The listing builds one solid part. Answer for the finished solid, in the listing's coordinates (mm). Face numbers are marked on the shaded views. A direction names the side the tool comes from. Round coordinates to 2 decimals unless told otherwise and drop trailing zeros. Write each loop counter-clockwise with the first axis right and the second up, starting at its lowest first coordinate (ties: lowest second). Pieces come first, ordered by that corner, then holes. Notation, with made-up numbers: (-4, -16) - (47, -16) arc R27 ccw to (47, 3) - close; hole circle Ø10 at (-1.5, 58.5). An arc over 180 degrees is marked (long way). Return JSON: item names as keys, results as strings. Group by question number.
Autodesk Inventor part; units mm, degrees
ref_plane "Work Plane4" through (55.733, 38.0112, -55.921) normal (0.7071, 0, -0.7071) x (0, -1, 0)
ref_plane "YZ Plane" through (0, 0, 0) normal (1, 0, 0) x (0, 1, 0)
ref_plane "XZ Plane" through (0, 0, 0) normal (0, 1, 0) x (-1, 0, 0)
sketch "Sketch1" plane through (0, 0, 0) normal (1, 0, 0) x (0, 1, 0)
  line L0 (0, 0) -> (155.1, 0)
  line L1 (155.1, 0) -> (155.1, -10)
  line L2 (0, -20) -> (0, 0)
  line L3 (155.1, -10) -> (101.6, -10)
  line L4 (101.6, -10) -> (101.6, -20)
  line L5 (101.6, -20) -> (0, -20)
  dimension "d0" = 53.5
  dimension "d1" = 155.1
  dimension "d2" = 10
  dimension "d3" = 10
  dimension "d4" = 20
extrude "Extrusion1" add sketch "Sketch1" along normal blind 629.2342
chamfer "Chamfer1" distance 19.812 angle 45 1 edges at (629.2342, 50.8, -20)
chamfer "Chamfer2" distance 19.812 angle 45 1 edges at (0, 50.8, -20)
ref_plane "Work Plane4" through (55.733, 38.0112, -55.921) normal (0.7071, 0, -0.7071) x (0, -1, 0)
sketch "Sketch3" plane through (55.733, 38.0112, -55.921) normal (0.7071, 0, -0.7071) x (0, -1, 0)
  line L0 (-63.5888, 0) -> (-63.5888, -416.9174)
  line L1 (-63.5888, 0) -> (38.0112, 0)
  line L2 (-117.0888, -0.1329) -> (-117.0888, -445.0687)
  line L3 (-117.0888, -0.1329) -> (-14.7014, -0.1329)
  line L4 (38.0112, -0.1329) -> (-117.0888, -0.1329)
  dimension "d18" = 102.3874
hole "Hole1" at (55.827, 52.7126, -55.827) direction (-0.7071, 0, 0.7071) diameter 12.7 depth 127 tip angle 118
properties part number "SkinnySideWidthOutlet" material "Wood (Birch)"
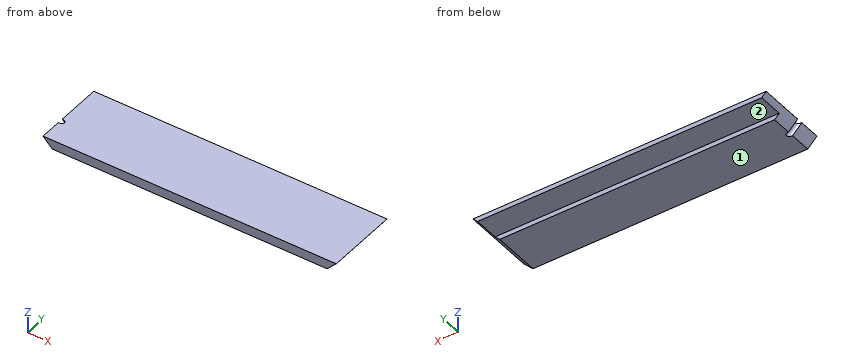
(1) Consider line 1 (Z direction, x = 411.5, y = 128); line 2 (Y direction, x = 178, z = -15.5); line 3 (X direction, y = 140, z = -3.25). Determine where each line is inside the solid, lowest interval first.
(2) For the marked faces 1 and 2, determine the directions among +Z, -Z, +X, -X, +Y, -Y from which every point of the face is accessible in a straight line to the end or side of a thin tool.
(3) Find section A-A (y = 18). Write down the section's boundary in (x, z).
(4) Find section B-B (x = 374). Write down the section's boundary in (y, z).
(5) Flat-ended cylindrical pins translate along their axes: pin 1 (3 mm diameter, centred on x = 397, y = 112.5, fed in from -Z); pin 2 (12 mm diameter, centred on y = 98.5, z = -13.5, fed in from +X); pin 3 (10 mm diameter, centred on y = 35, z = -16, fed in from +X). Find the tip coordinate at first contact, or state that the pin passes through.
Check sheet entries:
{
 "1": {"line 1": "z = -10 to 0", "line 2": "y = 0 to 101.6", "line 3": "x = 3.06 to 626.17"},
 "2": {"face 1": "-Z, +X, -X, +Y, -Y", "face 2": "-Z, +X, -X, +Y"},
 "3": {"outline": "(0, -0.19) - (19.81, -20) - (609.42, -20) - (629.23, -0.19) - (629.23, 0) - (0, 0) - close"},
 "4": {"outline": "(0, -20) - (101.6, -20) - (101.6, -10) - (155.1, -10) - (155.1, 0) - (0, 0) - close"},
 "5": {"pin 1": "stops at z = -10", "pin 2": "stops at x = 621.92", "pin 3": "stops at x = 618.42"}
}
